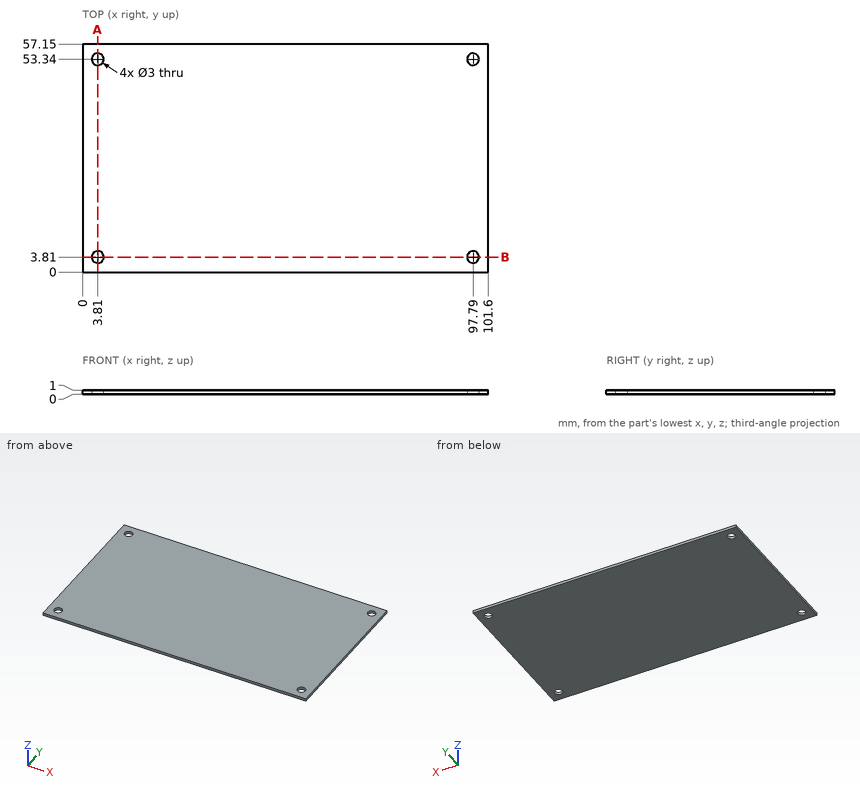
Source: three-view drawing plus pictorial views. Frame: mm from the lowest corner of the part. Coordinates: 2 decimals unless noted, no trailing zeros. Loops run counter-clockwise (first coordinate to the right, second up) from the corner with the lowest first, then second, coordinate; pieces in that order, holes last. Notation, with made-up numbers: (-26, 74.25) - (2, 74.25) arc R25 cw to (2, 95.25) - close; hole circle Ø8 at (12, 30.25). An arc over 180 degrees is marked (long way). Answer in a Markdown table with one row per item. Add a question column.
Item 1: Section query B-B on y = 3.81. Return the cut outline in (x, z).
Item 2: Section query A-A on x = 3.81. Return the cut outline in (y, z).
Item 3: Line query: line 1 along Y through (x, z) = (3.81, 0.3); line 2 along Y through (x, z) = (96.5, 0.8); line 3 along X through (y, z) = (5, 0.35). Output: solid intervals per line, ascending. Write a range as [from, to].
Item 4: Contact query for a flat-ended pin moving along its axis: P1, Ø1.8, axis at x = 3.81, y = 3.81, coming from the -Z side. Output: stop coordinate, or through.
Recorded:
| question | item | result |
|---|---|---|
| 1 | outline | (0, 0) - (2.31, 0) - (2.31, 1) - (0, 1) - close; (5.31, 0) - (96.29, 0) - (96.29, 1) - (5.31, 1) - close; (99.29, 0) - (101.6, 0) - (101.6, 1) - (99.29, 1) - close |
| 2 | outline | (0, 0) - (2.31, 0) - (2.31, 1) - (0, 1) - close; (5.31, 0) - (51.84, 0) - (51.84, 1) - (5.31, 1) - close; (54.84, 0) - (57.15, 0) - (57.15, 1) - (54.84, 1) - close |
| 3 | line 1 | [0, 2.31], [5.31, 51.84], [54.84, 57.15] |
| 3 | line 2 | [0, 3.04], [4.58, 52.57], [54.11, 57.15] |
| 3 | line 3 | [0, 2.9], [4.72, 96.88], [98.7, 101.6] |
| 4 | P1 | through |
